```python
from build123d import *

# Parameters (mm, degrees)
F0_W     = 118.0837154388
F0_H     = 70.6295147538
F1_DEPTH = 6.35
F2_R     = 7.62
F4_DEPTH = 25.4
F6_DEPTH = 50.8


with BuildPart() as f1:
    # F0 (on Top) → F1 (new body)
    with BuildSketch(Plane.XY):
        Rectangle(F0_W, F0_H)
    extrude(amount=F1_DEPTH)

    # F2
    f2_edges = [f1.edges().sort_by_distance(p)[0] for p in [
        (-59.041858, 35.314757, 3.175),
        (59.041858, 35.314757, 3.175),
    ]]
    fillet(f2_edges, radius=F2_R)

    # F3 (on face) → F4 (join)
    with BuildSketch(Plane.XY.offset(6.35)):
        with BuildLine():
            Line((-42.4880945322, 0), (-42.4880945322, -35.3147573769))
            Line((-42.4880945322, -35.3147573769), (-36.9701385498, -35.3147573769))
            Line((-36.9701385498, -35.3147573769), (-36.9701385498, -18.2091724128))
            Line((-36.9701385498, -18.2091724128), (34.7629673779, -18.2091724128))
            Line((34.7629673779, -18.2091724128), (34.7629673779, -35.3147573769))
            Line((34.7629673779, -35.3147573769), (43.0398620665, -35.3147573769))
            Line((43.0398620665, -35.3147573769), (43.0398620665, 0))
            ThreePointArc((43.0398620665, 0), (36.6044160593, 0.4599269685), (33.5122679292, 6.1225339714))
            Line((33.5122679292, 6.1225339714), (33.5122679292, 35.3147573769))
            Line((33.5122679292, 35.3147573769), (-32.6155844176, 35.3147573769))
            Line((-32.6155844176, 35.3147573769), (-32.6155844176, 5.9529215684))
            ThreePointArc((-32.6155844176, 5.9529215684), (-35.8708933771, 0.1887275405), (-42.4880945322, 0))
        make_face()
    extrude(amount=F4_DEPTH)

    # F5 (on face) → F6 (cut)
    with BuildSketch(Plane.XY.offset(31.75)):
        with BuildLine():
            ThreePointArc((-28.8878973408, 35.3147573769), (0.4483417558, 5.9785182804), (29.7845808524, 35.3147573769))
            Line((29.7845808524, 35.3147573769), (-28.8878973408, 35.3147573769))
        make_face()
    extrude(amount=-F6_DEPTH, mode=Mode.SUBTRACT)


solid = f1.part
```
Geometry: final body of the model. Coordinates: model frame, mm. A direction names the side the tool comes from. Round coordinates to 2 decimals unless told otherwise and drop trailing zeros. Write each loop counter-clockwise with the first axis right and the second up, starting at its lowest first coordinate (ties: lowest second). Pieces come first, ordered by that corner, then holes.
Item 1: Set-up query: faces 5 (the face through (33.512, 21, 19)), 6 (the face through (34.763, -27, 19)), 7 (the face through (43.04, -18, 19)). Return all of +Z, -Z, +X, -X, +Y, -Y with unobstructed straight access to the full face (end or side cutting, diameter ignored); none if empty.
Item 2: Pin query (flat end, axial travel): P1, Ø19, axis at y = -25, z = 23, coming from the +X side; P2, Ø5, axis at x = -16.5, y = -30.5, coming from the +Z side; P3, Ø8, axis at x = 14, z = 18.5, coming from the -Y side; P4, Ø8, axis at x = -1, y = 13.5, coming from the -Z side. Return the tip coordinate at first contact, or that it passes through.
Item 3: Material intervals for L1, parallel to Z at x = 37, y = 1; L2, parallel to Y at x = 32, z = 17; L3, parallel to X at y = -13.5, z = 12, sorted ascending.
Item 4: Section query D-D (x = 10.5). Return loops of the section in (y, z), plus the area to 3 significant figures.
Item 5: Mould query, pull axis X, two halves, no side actions, for faces 1 (the face through (0, -7, 31.75)), 2 (the face through (36.7, 0.4, 18.9)), 3 (the face through (-35.79, 0.24, 18.87)), 4 (the face through (56.87, 33.02, 3.22)). Classes: +X half, -X half, draft (parallel to the pull), parting line (faces both ways), or undercut.
Item 6: Section query A-A (y = 19.5). Return loops of the section in (x, z), plus the area to 3 significant figures.
Item 7: Section query B-B (y = -6.5). Return loops of the section in (x, z).
Completed:
1. face 5: +Z, +X, +Y
1. face 6: +Z, -Y
1. face 7: +Z, +X, +Y, -Y
2. P1: stops at x = 43.04
2. P2: stops at z = 6.35
2. P3: stops at y = -18.21
2. P4: passes through
3. L1: z = 0 to 6.35
3. L2: y = -18.21 to 35.31
3. L3: x = -42.49 to 43.04
4. outline: (-35.31, 0) - (7.75, 0) - (7.75, 31.75) - (-18.21, 31.75) - (-18.21, 6.35) - (-35.31, 6.35) - close
4. area: 933 mm2
5. face 1: draft
5. face 2: undercut
5. face 3: undercut
5. face 4: +X half
6. outline: (-59.04, 0) - (-24.26, 0) - (-24.26, 31.75) - (-32.62, 31.75) - (-32.62, 6.35) - (-59.04, 6.35) - close; (25.16, 0) - (59.04, 0) - (59.04, 6.35) - (33.51, 6.35) - (33.51, 31.75) - (25.16, 31.75) - close
6. area: 860 mm2
7. outline: (-59.04, 0) - (59.04, 0) - (59.04, 6.35) - (43.04, 6.35) - (43.04, 31.75) - (-42.49, 31.75) - (-42.49, 6.35) - (-59.04, 6.35) - close
